Verification items for the finished model (mm, model axes). Face numbers are marked on the shaded views. A direction names the side the tool comes from. Coordinates: 2 decimals unless noted, no trailing zeros. Order: outer loops, then holes, each group sorted by start corner. A loop starts at its lowest first (then second) coordinate and runs counter-clockwise, first axis right, second up. Notation, with made-up numbers: (84.25, -34.5) -> (118.25, -34.5) arc R18 cw to (118.25, -11.5) -> close; hole circle Ø3 at (-22, -23.5). An arc over 180 degrees is marked (long way). Use CSV: the item, a comma, the result in double quotes. Start each with the question number.
1) Go/stop test with flat-tipped pins: pin 1 (1 mm diameter, centred on x = 0.5, z = 0.5, fed in from +Y); pin 2 (1.5 mm diameter, centred on y = 6, z = 1, fed in from +X); pin 3 (2 mm diameter, centred on x = -1, z = 1.5, fed in from +Y); pin 4 (1.5 mm diameter, centred on y = 2.5, z = 2.5, fed in from +X). Record where each tip stops, or that it passes through.
2) Tool access check on the marked faces 1 and 2. Record the directions out of +Z, -Z, +X, -X, +Y, -Y that give a thin tool (end or side, any length) a straight path to the whole face; none if there is none.
3) Sectioned sample at A-A on z = 3. Record the boundary of the cut face in (x, y), then the cut area to 4 significant figures.
4) Scan lines: line 1 along X through (y, z) = (4, 0); line 2 along X through (y, z) = (6.85, 0). Record each from-to range of solid material in increasing order.
5) Sectioned sample at B-B on x = 0. Record the boundary of the cut face in (y, z), then the cut area to 4 significant figures.
6) Sectioned sample at C-C on y = 6. Record the boundary of the cut face in (x, z), then the cut area to 3 significant figures.
7) Sectioned sample at D-D on z = 0. Record the boundary of the cut face in (x, y).
8) Release check for a two-part mould opening along X. For the marked faces 3, 4 and 5 record: released by +X, released by -X, zero draft, split by the parting line, or undercut.
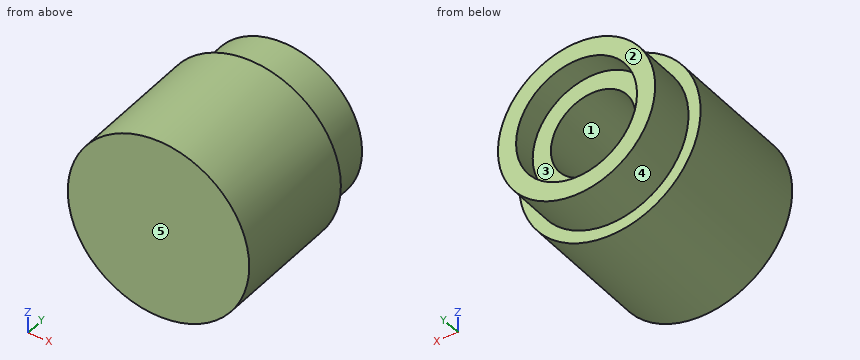
from build123d import *

# Parameters (mm, degrees)
SKETCH1_R           = 3.75
BOSS_EXTRUDE1_DEPTH = 7.5
SKETCH4_R           = 3.75
SKETCH4_R_2         = 3.25
CUT_EXTRUDE1_DEPTH  = 2
SKETCH5_R           = 1.75
CUT_EXTRUDE2_DEPTH  = 7
SKETCH6_R           = 2.5
CUT_EXTRUDE3_DEPTH  = 1


with BuildPart() as part:
    # Sketch1 → Boss-Extrude1 (new body)
    with BuildSketch(Plane(origin=(0, 0, 0), x_dir=(1, 0, 0), z_dir=(0, 1, 0))):
        Circle(SKETCH1_R)
    extrude(amount=BOSS_EXTRUDE1_DEPTH)

    # Sketch4 → Cut-Extrude1 (cut)
    with BuildSketch(Plane(origin=(0, 7.5, 0), x_dir=(1, 0, 0), z_dir=(0, 1, 0))):
        Circle(SKETCH4_R)
        Circle(SKETCH4_R_2, mode=Mode.SUBTRACT)
    extrude(amount=-CUT_EXTRUDE1_DEPTH, mode=Mode.SUBTRACT)

    # Sketch5 → Cut-Extrude2 (cut)
    with BuildSketch(Plane(origin=(0, 7.5, 0), x_dir=(1, 0, 0), z_dir=(0, 1, 0))):
        Circle(SKETCH5_R)
    extrude(amount=-CUT_EXTRUDE2_DEPTH, mode=Mode.SUBTRACT)

    # Sketch6 → Cut-Extrude3 (cut)
    with BuildSketch(Plane(origin=(0, 7.5, 0), x_dir=(1, 0, 0), z_dir=(0, 1, 0))):
        Circle(SKETCH6_R)
    extrude(amount=-CUT_EXTRUDE3_DEPTH, mode=Mode.SUBTRACT)


solid = part.part
Answers follow:
1,pin 1,"stops at y = 0.5"
1,pin 2,"stops at x = 3.72"
1,pin 3,"stops at y = 7.5"
1,pin 4,"stops at x = 3.32"
2,face 1,"+Y"
2,face 2,"+Z, -Z, +X, -X, +Y"
3,outline,"(-2.25, 0) -> (2.25, 0) -> (2.25, 5.5) -> (1.25, 5.5) -> (1.25, 7.5) -> (-1.25, 7.5) -> (-1.25, 5.5) -> (-2.25, 5.5) -> close"
3,area,"29.75 mm²"
4,line 1,"x = -3.75 to -1.75, 1.75 to 3.75"
4,line 2,"x = -3.25 to -2.5, 2.5 to 3.25"
5,outline,"(0, -3.75) -> (5.5, -3.75) -> (5.5, -3.25) -> (7.5, -3.25) -> (7.5, -2.5) -> (6.5, -2.5) -> (6.5, -1.75) -> (0.5, -1.75) -> (0.5, 1.75) -> (6.5, 1.75) -> (6.5, 2.5) -> (7.5, 2.5) -> (7.5, 3.25) -> (5.5, 3.25) -> (5.5, 3.75) -> (0, 3.75) -> close"
5,area,"28.25 mm²"
6,outline,"circle Ø6.5 at (0, 0); hole circle Ø3.5 at (0, 0)"
6,area,"23.6 mm²"
7,outline,"(-3.75, 0) -> (3.75, 0) -> (3.75, 5.5) -> (3.25, 5.5) -> (3.25, 7.5) -> (2.5, 7.5) -> (2.5, 6.5) -> (1.75, 6.5) -> (1.75, 0.5) -> (-1.75, 0.5) -> (-1.75, 6.5) -> (-2.5, 6.5) -> (-2.5, 7.5) -> (-3.25, 7.5) -> (-3.25, 5.5) -> (-3.75, 5.5) -> close"
8,face 3,"undercut"
8,face 4,"split by the parting line"
8,face 5,"zero draft"
